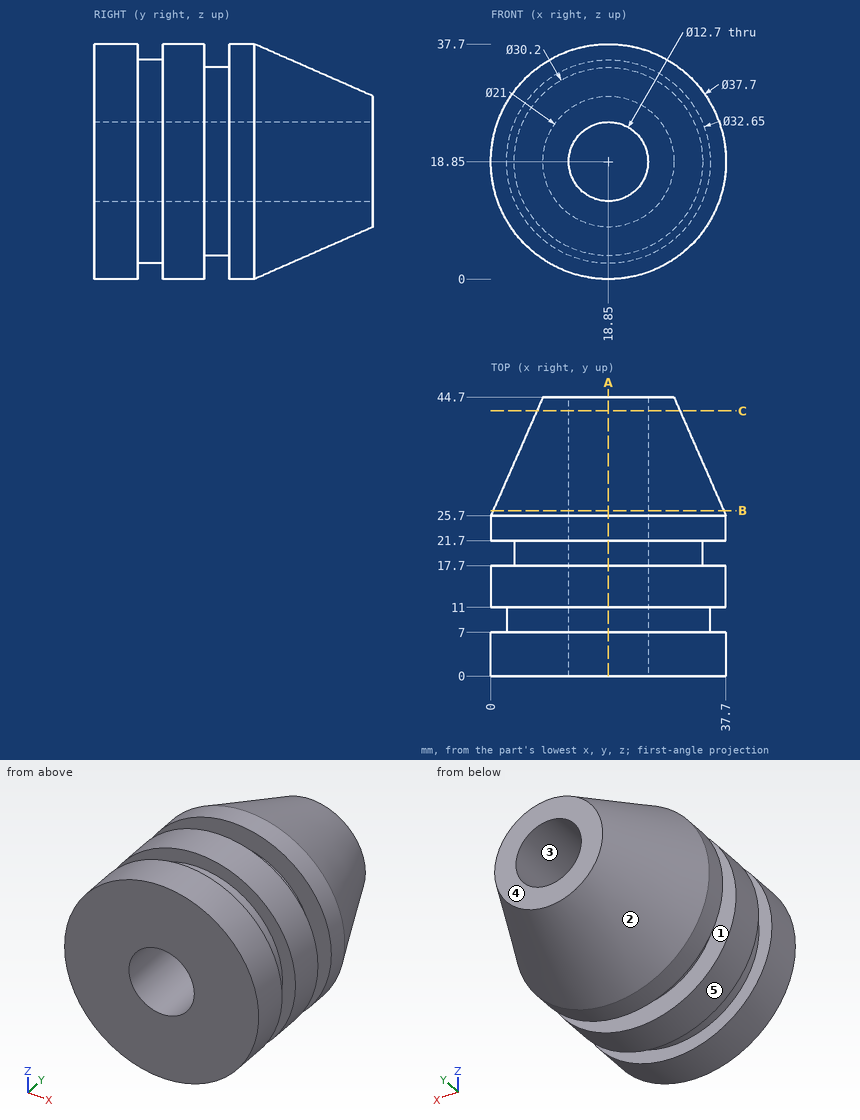
Answer from the drawing. Dimensions are ordinates in mm from the lowest x, y and z of the part. A direction names the side the tool comes from. Round coordinates to 2 decimals unless told otherwise and drop trailing zeros. Loops run counter-clockwise (first coordinate to the right, second up) from the corner with the lowest first, then second, coordinate; pieces in that order, holes last.
(1) For the marked faces 1 and 2, determine the directions among +Z, -Z, +X, -X, +Y, -Y from which every point of the face is accessible in a straight line to the end or side of a thin tool.
Computed values:
face 1: none
face 2: +Y
(2) The mould has two halves that part along X. Classify the marked faces 3, 4 and 5: pulls with the +X half, pulls with the -X half, needs draft (parallel to the pull), parting line crosses it, or undercut.
Computed values:
face 3: undercut
face 4: needs draft
face 5: parting line crosses it
(3) Find the intervals of material crossed by L1, parallel to Z at x = 18.85, y = 14.5; L2, parallel to Z at x = 18.85, y = 19; L3, parallel to Y at x = 36, z = 20, in increasing order.
Computed values:
L1: z = 0 to 12.5, 25.2 to 37.7
L2: z = 3.75 to 12.5, 25.2 to 33.95
L3: y = 0 to 7, 11 to 17.7, 21.7 to 29.48
(4) The part is cut by section B-B, the plane y = 26.5. Give the vertices of the cut face in (x, z).
Computed values:
outline: circle Ø37 at (18.85, 18.85); hole circle Ø12.7 at (18.85, 18.85)
(5) Each of these flat-tipped pins is pushed along its axis until it touches: P1, Ø1.5, axis at y = 21, z = 19.5, coming from the -X side; P2, Ø8, axis at x = 20.5, y = 33, coming from the -Z side; P3, Ø2, axis at y = 37.5, z = 19, coming from the -X side; P4, Ø11.5, axis at x = 25, z = 20, coming from the -Y side. Where does it stop, or does it pass through?
Computed values:
P1: stops at x = 0
P2: stops at z = 1.5
P3: stops at x = 4.75
P4: stops at y = 0
(6) The part is cut by section C-C, the plane y = 42.5. Give the vertices of the cut face in (x, z).
Computed values:
outline: circle Ø22.93 at (18.85, 18.85); hole circle Ø12.7 at (18.85, 18.85)
(7) The part is cut by section A-A, the plane x = 18.85. Give the vertices of the cut face in (y, z) (3 decimals).
Computed values:
outline: (0, 0) - (7, 0) - (7, 2.525) - (11, 2.525) - (11, 0) - (17.7, 0) - (17.7, 3.75) - (21.7, 3.75) - (21.7, 0) - (25.7, 0) - (44.7, 8.35) - (44.7, 12.5) - (0, 12.5) - close; (0, 25.2) - (44.7, 25.2) - (44.7, 29.35) - (25.7, 37.7) - (21.7, 37.7) - (21.7, 33.95) - (17.7, 33.95) - (17.7, 37.7) - (11, 37.7) - (11, 35.175) - (7, 35.175) - (7, 37.7) - (0, 37.7) - close
